```python
from build123d import *
from OCP.BRepAlgoAPI import BRepAlgoAPI_Cut
from OCP.TopTools import TopTools_ListOfShape

# Parameters (mm, degrees)
SKETCH1_W           = 21
SKETCH1_H           = 31
BOSS_EXTRUDE1_DEPTH = 30
SKETCH2_W           = 21
SKETCH2_H           = 17.936176812
BOSS_EXTRUDE2_DEPTH = 45
SKETCH6_R           = 2
CUT_EXTRUDE1_DEPTH  = 30
SKETCH8_W           = 62.569062922
SKETCH8_H           = 62.569062922
SKETCH8_R           = 2.5
BOSS_EXTRUDE6_DEPTH = 6
FILLET1_R           = 20
FILLET2_R           = 20
FILLET3_START       = -10.5
FILLET3_DEPTH       = 21
FILLET3_START_2     = -38.284535634
FILLET3_2_DEPTH     = 46.220712446
FILLET3_START_3     = -22
FILLET3_3_DEPTH     = 43
SKETCH9_W           = 5.5
SKETCH9_H           = 4.5
CUT_EXTRUDE2_DEPTH  = 25
SKETCH10_W          = 4.5
SKETCH10_H          = 3.134245462
CUT_EXTRUDE3_DEPTH  = 25


with BuildPart() as part:
    # Sketch1 → Boss-Extrude1 (new body)
    with BuildSketch(Plane.XY):
        Rectangle(SKETCH1_W, SKETCH1_H)
    extrude(amount=-BOSS_EXTRUDE1_DEPTH)

    # Sketch2 → Boss-Extrude2 (add)
    with BuildSketch(Plane.XZ.offset(15.5)):
        with Locations((0, -21.031911594)):
            Rectangle(SKETCH2_W, SKETCH2_H)
    extrude(amount=BOSS_EXTRUDE2_DEPTH)

    # Sketch6 → Cut-Extrude1 (cut)
    with BuildSketch(Plane.XY):
        with Locations((5.5, 5.5)):
            Circle(SKETCH6_R)
        with Locations((5.5, -5.5)):
            Circle(SKETCH6_R)
        with Locations((-5.5, -5.5)):
            Circle(SKETCH6_R)
        with Locations((-5.5, 5.5)):
            Circle(SKETCH6_R)
    extrude(amount=-CUT_EXTRUDE1_DEPTH, mode=Mode.SUBTRACT)

    # Sketch8 → Boss-Extrude6 (add)
    with BuildSketch(Plane.XZ.offset(60.5)):
        with Locations((0, -7)):
            Rectangle(SKETCH8_W, SKETCH8_H)
        with Locations(Location((23, 16, 0), (0, 0, 270))):
            Circle(SKETCH8_R, mode=Mode.SUBTRACT)
        with Locations(Location((23, -30, 0), (0, 0, 270))):
            Circle(SKETCH8_R, mode=Mode.SUBTRACT)
        with Locations(Location((-23, -30, 0), (0, 0, 270))):
            Circle(SKETCH8_R, mode=Mode.SUBTRACT)
        with Locations(Location((-23, 16, 0), (0, 0, 270))):
            Circle(SKETCH8_R, mode=Mode.SUBTRACT)
    extrude(amount=BOSS_EXTRUDE6_DEPTH)

    # Fillet1
    fillet1_edges = [part.edges().sort_by_distance(p)[0] for p in [
        (0, -60.5, -12.063823188),
    ]]
    fillet(fillet1_edges, radius=FILLET1_R)

    # Fillet2
    # the kernel refuses this fillet: 20 mm, written as the material it adds along each edge
    with BuildSketch(Plane(origin=(-10.5, -15.5, -12.063823188), x_dir=(0, 0, 1), z_dir=(1, 0, 0))) as fillet2_piece_1:
        with BuildLine():
            CenterArc((20, 18.358025428), FILLET2_R, 180, 66.621165334)
            Line((0, 18.358025428), (-0.4, 18.358025428))
            Line((-0.4, 18.358025428), (-0.4, 0))
            Line((-0.4, 0), (0, -0.4))
            ThreePointArc((0, -0.4), (6.031911594, -0.4), (11.905099651, -0.367160509))
            Line((11.905099651, -0.367160509), (12.063823188, 0))
        make_face()
    extrude(amount=21)


with BuildPart() as fillet3_tool:
    # Fillet3: read off the stored shape, not the designer's step
    # Fillet3 outline → Fillet3 (new body)
    with BuildSketch(Plane.YZ.offset(FILLET3_START)):
        with BuildLine():
            ThreePointArc((-60.5, -38.284531461), (-57.084283982, -32.34641635), (-50.648240376, -30))
            Line((-50.648240376, -30), (-60.5, -30))
            Line((-60.5, -30), (-60.5, -38.284531461))
        make_face()
    extrude(amount=FILLET3_DEPTH)


with BuildPart() as part_1:
    add(part.part)


with BuildPart() as part_2:
    # Fillet3: joined with fillet3_tool
    add(part_1.part.fuse(fillet3_tool.part, tol=0.00001))


with BuildPart() as fillet3_2_tool:
    # Fillet3 2 outline → Fillet3 2 (new body)
    with BuildSketch(Plane.XY.offset(FILLET3_START_2)):
        with BuildLine():
            Line((10.5, -50.5), (10.5, -60.5))
            Line((10.5, -60.5), (20.5, -60.5))
            ThreePointArc((20.5, -60.5), (13.428932188, -57.571067812), (10.5, -50.5))
        make_face()
        with BuildLine():
            ThreePointArc((-10.5, -50.5), (-13.428932188, -57.571067812), (-20.5, -60.5))
            Line((-20.5, -60.5), (-10.5, -60.5))
            Line((-10.5, -60.5), (-10.5, -50.5))
        make_face()
    extrude(amount=FILLET3_2_DEPTH)


with BuildPart() as part_3:
    add(part_2.part)


with BuildPart() as part_4:
    # Fillet3 2: joined with fillet3_2_tool
    add(part_3.part.fuse(fillet3_2_tool.part, tol=0.00001))


with BuildPart() as fillet3_3_tool:
    # Fillet3 3 outline → Fillet3 3 (new body)
    with BuildSketch(Plane.YZ.offset(FILLET3_START_3)):
        with BuildLine():
            ThreePointArc((-50.648240376, -30), (-57.084283982, -32.34641635), (-60.5, -38.284531461))
            Line((-60.5, -38.284531461), (-50.5, -38.284535634))
            Line((-50.5, -38.284535634), (-50.5, -30))
            Line((-50.5, -30), (-50.648240376, -30))
        make_face()
        with BuildLine():
            Line((-50.5, 7.936176812), (-60.5, 7.936176812))
            ThreePointArc((-60.5, 7.936176812), (-57.820508076, -2.063823188), (-50.5, -9.384331263))
            Line((-50.5, -9.384331263), (-50.5, 7.936176812))
        make_face()
    extrude(amount=FILLET3_3_DEPTH)


with BuildPart() as part_5:
    add(part_4.part)

    # Fillet3 3: cut by fillet3_3_tool, with a tolerance
    fillet3_3_stock = TopTools_ListOfShape()
    fillet3_3_stock.Append(part_5.part.wrapped)
    fillet3_3_tools = TopTools_ListOfShape()
    fillet3_3_tools.Append(fillet3_3_tool.part.wrapped)
    fillet3_3_cut = BRepAlgoAPI_Cut()
    fillet3_3_cut.SetArguments(fillet3_3_stock)
    fillet3_3_cut.SetTools(fillet3_3_tools)
    fillet3_3_cut.SetFuzzyValue(0.00001)
    fillet3_3_cut.Build()
    add(Compound.cast(fillet3_3_cut.Shape()).solids(), mode=Mode.REPLACE)

    # Sketch9 → Cut-Extrude2 (cut)
    with BuildSketch(Plane(origin=(0, 15.5, 0), x_dir=(1, 0, 0), z_dir=(0, 1, 0))):
        with Locations((-5.5, 12.25)):
            Rectangle(SKETCH9_W, SKETCH9_H)
        with Locations((5.5, 12.25)):
            Rectangle(SKETCH9_W, SKETCH9_H)
    extrude(amount=-CUT_EXTRUDE2_DEPTH, mode=Mode.SUBTRACT)

    # Sketch10 → Cut-Extrude3 (cut)
    with BuildSketch(Plane.ZY.offset(10.5)):
        with Locations((-12.25, -11.067122731)):
            Rectangle(SKETCH10_W, SKETCH10_H)
    extrude(amount=-CUT_EXTRUDE3_DEPTH, mode=Mode.SUBTRACT)


solid = part_5.part
```
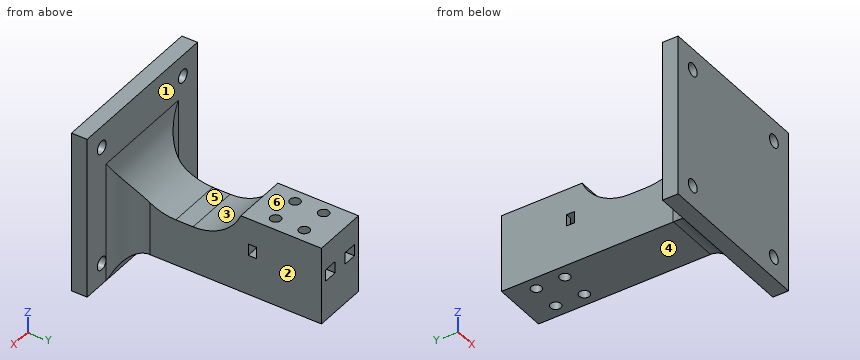
The model under review builds one solid part; all positions refer to its coordinate system, in mm. Face numbers are marked on the shaded views. A direction names the side the tool comes from. Coordinates: 2 decimals unless noted, no trailing zeros. Order: outer loops, then holes, each group sorted by start corner. A loop starts at its lowest first (then second) coordinate and runs counter-clockwise, first axis right, second up. Notation, with made-up numbers: (-22.5, -2.5) -> (10.5, -2.5) arc R34 cw to (10.5, 31.5) -> close; hole circle Ø1 at (30, -37.5). An arc over 180 degrees is marked (long way). Answer in a Markdown table with one row per item. Add a question column.
Item 1: We need section A-A on z = 16. Write out the cut boundary in (x, y), plus the area to 3 significant figures.
Item 2: To check wall thickness, follow probe 1 along Z at (x, y) = (-4, 11.5); probe 2 along Y at (x, z) = (-5, -19); probe 3 along X at (y, z) = (-49, -16). State the ranges of each line that lie inside material, in increasing order.
Item 3: Machinability: for the marked faces 4, 5 and 6, which of the approach directions +Z, -Z, +X, -X, +Y, -Y give a long, thin tool a straight path to every point of the face, cutting with its end or side? Answer none if there is none.
Item 4: We need section D-D on z = -25. Write out the cut boundary in (x, y).
Item 5: Mouldability with a two-part tool opening along Y and no side actions: class the marked faces 1, 2 and 3 as +Y half, -Y half, draft (parallel to the pull), parting line (faces both ways), or undercut.
Item 6: We need section C-C on x = -5.5. Give the number of separate pieces and of enclosed holes in the cut face, plus the area to 3 significant figures.
Item 7: Clearance check with flat-ended pins moving along their axes: pin 1 (2.5 mm diameter, centred on x = 5.5, y = -5.5, fed in from +Z); pin 2 (3 mm diameter, centred on x = 19, z = 16.5, fed in from +Y); pin 3 (5 mm diameter, centred on x = -5.5, y = -5.5, fed in from +Z); pin 4 (1 mm diameter, centred on x = 6, z = 7, fed in from +Y). State where each tip first meets the part, or that it passes through.
Item 8: We need section B-B on y = -5.5. Write out the cut boundary in (x, z), plus the area to 4 significant figures.
Final values:
| question | item | result |
|---|---|---|
| 1 | outline | (-31.28, -66.5) -> (-25.5, -66.5) -> (-25.5, -60.5) -> (-31.28, -60.5) -> close; (-20.5, -66.5) -> (20.5, -66.5) -> (20.5, -60.5) -> (-20.5, -60.5) -> close; (25.5, -66.5) -> (31.28, -66.5) -> (31.28, -60.5) -> (25.5, -60.5) -> close |
| 1 | area | 315 mm2 |
| 2 | probe 1 | z = -30 to -14.5, -10 to 0 |
| 2 | probe 2 | y = -66.5 to -7.44, -3.56 to 3.56, 7.44 to 15.5 |
| 2 | probe 3 | x = -10.5 to 10.5 |
| 3 | face 4 | -Z, +X, -X, +Y |
| 3 | face 5 | +Z, +X, -X |
| 3 | face 6 | +Z, +X, -X, +Y |
| 4 | outline | (-31.28, -66.5) -> (31.28, -66.5) -> (31.28, -60.5) -> (20.5, -60.5) arc R10 cw to (10.5, -50.5) -> (10.5, 15.5) -> (-10.5, 15.5) -> (-10.5, -50.5) arc R10 cw to (-20.5, -60.5) -> (-31.28, -60.5) -> close; hole circle Ø4 at (-5.5, -5.5); hole circle Ø4 at (-5.5, 5.5); hole circle Ø4 at (5.5, -5.5); hole circle Ø4 at (5.5, 5.5) |
| 5 | face 1 | +Y half |
| 5 | face 2 | draft |
| 5 | face 3 | undercut |
| 6 | separate pieces | 5 |
| 6 | enclosed holes | 0 |
| 6 | area | 1,950 mm2 |
| 7 | pin 1 | passes through |
| 7 | pin 2 | stops at y = -60.5 |
| 7 | pin 3 | stops at z = 0 |
| 7 | pin 4 | stops at y = -60.45 |
| 8 | outline | (-10.5, -30) -> (-7.5, -30) -> (-7.5, -14.5) -> (-8.25, -14.5) -> (-8.25, -10) -> (-7.5, -10) -> (-7.5, 0) -> (-10.5, 0) -> close; (-3.5, -30) -> (3.5, -30) -> (3.5, -14.5) -> (2.75, -14.5) -> (2.75, -10) -> (3.5, -10) -> (3.5, 0) -> (-3.5, 0) -> (-3.5, -10) -> (-2.75, -10) -> (-2.75, -14.5) -> (-3.5, -14.5) -> close; (7.5, -30) -> (10.5, -30) -> (10.5, 0) -> (7.5, 0) -> (7.5, -10) -> (8.25, -10) -> (8.25, -14.5) -> (7.5, -14.5) -> close |
| 8 | area | 376.5 mm2 |
